Design review of the part built by this model. Coordinates are the model's own, in mm. A direction names the side the tool comes from. Coordinates: 2 decimals unless noted, no trailing zeros. Loops run counter-clockwise (first coordinate to the right, second up) from the corner with the lowest first, then second, coordinate; pieces in that order, holes last. Notation, with made-up numbers: (-0.5, 25.25) -> (35.5, 25.25) arc R17 cw to (35.5, 54.25) -> close; hole circle Ø9 at (79, 35). An arc over 180 degrees is marked (long way). Use one line per item in the form item = value. Start each with the question number.
1. Consider section A-A (z = 27.5). State the section outline as (x, y) points.
2. Wall thickness on line 1 (Y direction, x = 23.58, z = 1.05); line 2 (X direction, y = -23, z = 3); line 3 (Y direction, x = -23, z = 2): over which ranges is each line inside the solid? List them lowest first. Write a range as from..to.
3. For pin 1 (1 mm diameter, centred on x = 8.5, z = 51.5, fed in from -Y); pin 2 (22.5 mm diameter, centred on x = 11.5, y = -16, fed in from +Z); pin 3 (8 mm diameter, centred on x = -6.5, y = 8.5, fed in from -Z); pin 4 (5 mm diameter, centred on x = 9, z = 34.5, fed in from +Y), all flat-tipped, find the tip position at first contact; note any pin that passes through.
4. Machinability: for faces 5 (the face through (26.055, 24.41, 2.381)), 6 (the face through (-15.12, -11.59, -0.77)), 7 (the face through (-21, 21, 4.83)), 8 (the face through (13.01, -25.02, 26.97)), which of the approach directions +Z, -Z, +X, -X, +Y, -Y give a long, thin tool a straight path to every point of the face, cutting with its end or side? Answer none if there is none.
5. Consider section B-B (z = -7). State the section outline as (x, y) points (3 decimals).
6. The part is to be moulded in two halves that separate along X. For faces 1 (the face through (-25.643, -25.162, 2.381)), 2 (the face through (-0.69, -3.1, 59.38)), 3 (the face through (21.517, -25.162, 2.381)), 4 (the face through (0, 0, -15.77)), say which applies: released by +X, released by -X, zero draft, split by the parting line, or undercut.
from build123d import *

# Parameters (mm, degrees)
ESBO_O1_R                = 2.6
ESBO_O1_R_2              = 3.175
RESSALTO_EXTRUS_O1_DEPTH = 4.83
RESSALTO_EXTRUS_O2_START = -1.52
ESBO_O2_R                = 19.05
ESBO_O2_R_2              = 3.175
RESSALTO_EXTRUS_O2_DEPTH = 1.52
ESBO_O3_R                = 28.2
RESSALTO_EXTRUS_O3_DEPTH = 45.4
RESSALTO_EXTRUS_O4_START = 20.6
ESBO_O4_R                = 3.175
RESSALTO_EXTRUS_O4_DEPTH = 20.6
FILETE1_R                = 0.5
ESBO_O5_R                = 3.175
RESSALTO_EXTRUS_O5_DEPTH = 19.05
FILETE2_R                = 0.5
FILETE3_R                = 0.5


with BuildPart() as part:
    # Esboço1 → Ressalto-extrusão1 (new body)
    with BuildSketch(Plane.XY):
        with BuildLine():
            Line((-23.58, -28.2), (23.58, -28.2))
            ThreePointArc((23.58, -28.2), (26.846833329, -26.846833329), (28.2, -23.58))
            Line((28.2, -23.58), (28.2, 23.58))
            ThreePointArc((28.2, 23.58), (26.846833329, 26.846833329), (23.58, 28.2))
            Line((23.58, 28.2), (-23.58, 28.2))
            ThreePointArc((-23.58, 28.2), (-26.846833329, 26.846833329), (-28.2, 23.58))
            Line((-28.2, 23.58), (-28.2, -23.58))
            ThreePointArc((-28.2, -23.58), (-26.846833329, -26.846833329), (-23.58, -28.2))
        make_face()
        with Locations((-23.57, 23.57)):
            Circle(ESBO_O1_R, mode=Mode.SUBTRACT)
        with Locations((23.575450692, 23.629295607)):
            Circle(ESBO_O1_R, mode=Mode.SUBTRACT)
        with Locations((23.58, -23.58)):
            Circle(ESBO_O1_R, mode=Mode.SUBTRACT)
        with Locations((-23.58, -23.58)):
            Circle(ESBO_O1_R, mode=Mode.SUBTRACT)
        Circle(ESBO_O1_R_2, mode=Mode.SUBTRACT)
    extrude(amount=RESSALTO_EXTRUS_O1_DEPTH)

    # Esboço2 → Ressalto-extrusão2 (add)
    with BuildSketch(Plane.XY.offset(RESSALTO_EXTRUS_O2_START)):
        Circle(ESBO_O2_R)
        Circle(ESBO_O2_R_2, mode=Mode.SUBTRACT)
    extrude(amount=RESSALTO_EXTRUS_O2_DEPTH)

    # Esboço3 → Ressalto-extrusão3 (add)
    with BuildSketch(Plane.XY.offset(4.83)):
        Circle(ESBO_O3_R)
    extrude(amount=RESSALTO_EXTRUS_O3_DEPTH)

    # Esboço4 → Ressalto-extrusão4 (add)
    with BuildSketch(Plane(origin=(0, 0, 4.83), x_dir=(-1, 0, 0), z_dir=(0, 0, -1)).offset(RESSALTO_EXTRUS_O4_START)):
        with Locations(Location((0, 0, 0), (0, 0, 180))):
            Circle(ESBO_O4_R)
    extrude(amount=-RESSALTO_EXTRUS_O4_DEPTH)

    # Filete1
    filete1_edges = [part.edges().sort_by_distance(p)[0] for p in [
        (-3.175, 0, -15.77),
    ]]
    fillet(filete1_edges, radius=FILETE1_R)

    # Esboço5 → Ressalto-extrusão5 (add)
    with BuildSketch(Plane.XY.offset(50.23)):
        Circle(ESBO_O5_R)
    extrude(amount=RESSALTO_EXTRUS_O5_DEPTH)

    # Filete2
    filete2_edges = [part.edges().sort_by_distance(p)[0] for p in [
        (-3.175, 0, 69.28),
    ]]
    fillet(filete2_edges, radius=FILETE2_R)

    # Filete3
    filete3_edges = [part.edges().sort_by_distance(p)[0] for p in [
        (-28.2, 0, 50.23),
    ]]
    fillet(filete3_edges, radius=FILETE3_R)


solid = part.part
Geometry check:
q1.outline = circle Ø56.4 at (0, 0)
q2.line_1 = -28.2..-26.18, -20.98..21.03, 26.23..28.2
q2.line_2 = -28.2..-26.11, -21.05..21.05, 26.11..28.2
q2.line_3 = -28.2..-26.11, -21.05..21.03, 26.11..28.2
q3.pin_1 = through
q3.pin_2 = 50.23
q3.pin_3 = -1.52
q3.pin_4 = 27.44
q4.face_5 = +Z, -Z
q4.face_6 = -Z
q4.face_7 = +Z, -X, +Y
q4.face_8 = +Z
q5.outline = circle Ø6.35 at (0, 0)
q6.face_1 = undercut
q6.face_2 = split by the parting line
q6.face_3 = undercut
q6.face_4 = zero draft
